Check sheet for the drawn part. Datum: minimum x, y, z corner. Units: mm. A direction names the side the tool comes from. Give positions to 0.01 mm unless a question says otherwise; leave off trailing zeros. Order: outer loops, then holes, each group sorted by start corner. A loop starts at its lowest first (then second) coordinate and runs counter-clockwise, first axis right, second up. Notation, with made-up numbers: (39, 83) -> (52, 83) arc R13 ccw to (52, 92) -> close; hole circle Ø10 at (12, 24). An arc over 180 degrees is marked (long way). One line per question, with ' | ' between items. Start each with the question number.
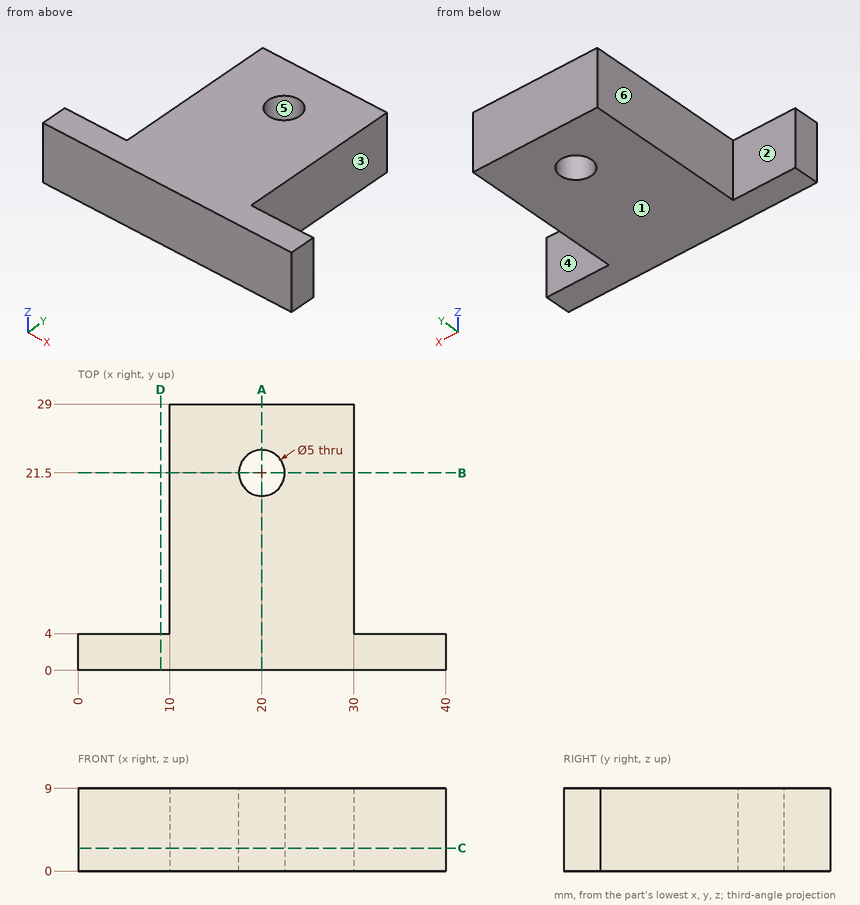
1. Go/stop test with flat-tipped pins: pin 1 (2.5 mm diameter, centred on y = 11.5, z = 4.5, fed in from -X); pin 2 (2 mm diameter, centred on x = 32, y = 7.5, fed in from -Z); pin 3 (4.5 mm diameter, centred on x = 36.5, z = 6, fed in from +Y); pin 4 (4 mm diameter, centred on y = 16, z = 5, fed in from +X). Record where each tip stops, or that it passes through.
2. Cross-section at D-D on x = 9. Record the boundary of the cut face in (y, z).
3. Mould release check, pull along X, two halves, no side actions. Record for the marked faces 4, 5 and 6: +X half, -X half, draft (parallel to the pull), parting line (faces both ways), or undercut.
4. Cross-section at A-A on x = 20. Record the boundary of the cut face in (y, z), and give its area (3 significant figures).
5. Scan lines: probe 1 along Y at (x, z) = (20, 2.5); probe 2 along X at (y, z) = (4.5, 8); probe 3 along Y at (x, z) = (20.5, 3). Record each from-to range of solid material in increasing order.
6. Tool access check on the marked faces 1, 2 and 3. Record the directions out of +Z, -Z, +X, -X, +Y, -Y that give a thin tool (end or side, any length) a straight path to the whole face; none if there is none.
7. Cross-section at C-C on z = 2.5. Record the boundary of the cut face in (x, y), and give its area (3 significant figures).
8. Cross-section at B-B on y = 21.5. Record the boundary of the cut face in (x, z).
Response values:
1) pin 1: stops at x = 10 | pin 2: passes through | pin 3: stops at y = 4 | pin 4: stops at x = 30
2) outline: (0, 0) -> (4, 0) -> (4, 9) -> (0, 9) -> close
3) face 4: draft | face 5: undercut | face 6: -X half
4) outline: (0, 0) -> (19, 0) -> (19, 9) -> (0, 9) -> close; (24, 0) -> (29, 0) -> (29, 9) -> (24, 9) -> close | area: 216 mm²
5) probe 1: y = 0 to 19, 24 to 29 | probe 2: x = 10 to 30 | probe 3: y = 0 to 19.05, 23.95 to 29
6) face 1: -Z, +X, -X, +Y, -Y | face 2: +Z, -Z, -X, +Y | face 3: +Z, -Z, +X, +Y
7) outline: (0, 0) -> (40, 0) -> (40, 4) -> (30, 4) -> (30, 29) -> (10, 29) -> (10, 4) -> (0, 4) -> close; hole circle Ø5 at (20, 21.5) | area: 640 mm²
8) outline: (10, 0) -> (17.5, 0) -> (17.5, 9) -> (10, 9) -> close; (22.5, 0) -> (30, 0) -> (30, 9) -> (22.5, 9) -> close
